```python
from build123d import *

# Parameters (mm, degrees)
BOSS_EXTRUDE1_DEPTH   = 10
M8_TAPPED_HOLE1_D     = 6.8
M8_TAPPED_HOLE1_DEPTH = 14
M8_TAPPED_HOLE1_TIP   = 2.042926105
M5_TAPPED_HOLE1_D     = 4.2
M5_TAPPED_HOLE1_DEPTH = 12
M5_TAPPED_HOLE1_TIP   = 1.2618073


with BuildPart() as part:
    # Sketch1 → Boss-Extrude1 (new, symmetric)
    with BuildSketch(Plane(origin=(0, 0, 0), x_dir=(0, 0, -1), z_dir=(1, 0, 0))):
        Polygon((12, 10), (-12, 10), (-12, 0), (-22, 0), (-22, 32), (22, 32), (22, 0), (12, 0), align=None)
    extrude(amount=BOSS_EXTRUDE1_DEPTH, both=True)

    # M8 Tapped Hole1
    with Locations(Plane(origin=(10, 0, 0), x_dir=(0, 0, -1), z_dir=(1, 0, 0))):
        with Locations((0, 18)):
            Hole(M8_TAPPED_HOLE1_D / 2, depth=M8_TAPPED_HOLE1_DEPTH)
            with Locations((0, 0, -(M8_TAPPED_HOLE1_DEPTH + M8_TAPPED_HOLE1_TIP / 2))):  # 118° drill point
                Cone(0, M8_TAPPED_HOLE1_D / 2, M8_TAPPED_HOLE1_TIP, mode=Mode.SUBTRACT)

    # M5 Tapped Hole1
    with Locations(Plane(origin=(0, 0, 0), x_dir=(-1, 0, 0), z_dir=(0, -1, 0))):
        with Locations((0, 17), (0, -17)):
            Hole(M5_TAPPED_HOLE1_D / 2, depth=M5_TAPPED_HOLE1_DEPTH)
            with Locations((0, 0, -(M5_TAPPED_HOLE1_DEPTH + M5_TAPPED_HOLE1_TIP / 2))):  # 118° drill point
                Cone(0, M5_TAPPED_HOLE1_D / 2, M5_TAPPED_HOLE1_TIP, mode=Mode.SUBTRACT)


solid = part.part
```
Input: part model. Units: mm. Frame: model coordinates. A direction names the side the tool comes from. Give positions to 0.01 mm unless a question says otherwise; leave off trailing zeros. Order: outer loops, then holes, each group sorted by start corner. A loop starts at its lowest first (then second) coordinate and runs counter-clockwise, first axis right, second up. Notation, with made-up numbers: M 16,23 L 54,23 A21 cw 54,43 Z; hole C 15.5,56 d2. An arc over 180 degrees is marked long. Return JSON: item names as keys, results as strings.
Item 1: Pull-direction query (Y, two-part tool) for faces 4 (the conical face through (-5.688, 18.498, -0.317)), 5 (the conical face through (-0.2, 13.04, -17.31)), 6 (the cylindrical face through (1.13, 6.08, -18.77)), 7 (the cylindrical face through (2.9, 14.68, -0.74)); classes: +Y half, -Y half, draft (parallel to the pull), parting line (faces both ways), or undercut.
Solutions:
{"face 4": "undercut", "face 5": "-Y half", "face 6": "draft", "face 7": "undercut"}
Item 2: Cut plane A-A (y = 7). Return loops of the section in (x, z).
Solutions:
{"outline": "M -10,-22 L 10,-22 L 10,-12 L -10,-12 Z; M -10,12 L 10,12 L 10,22 L -10,22 Z; hole C 0,-17 d4.2; hole C 0,17 d4.2"}
Item 3: Cut plane B-B (x = 6.5). Return loops of the section in (y, z), then the cut area to 3 significant figures.
Solutions:
{"outline": "M 0,-22 L 32,-22 L 32,22 L 0,22 L 0,12 L 10,12 L 10,-12 L 0,-12 Z; hole C 18,0 d6.8", "area": "1,130 mm^2"}
Item 4: Access query for faces 1 (the cylindrical face through (-0.273, 6.084, 14.918)), 2 (the flat face through (0, 32, 0)), 3 (the flat face through (0, 5, 12)). Directions: +Z, -Z, +X, -X, +Y, -Y. A direction counts if a zero-diameter tool reaches every point of the face in a straight line with its end or side. Return the directions, or none.
Solutions:
{"face 1": "-Y", "face 2": "+Z, -Z, +X, -X, +Y", "face 3": "+X, -X, -Y"}
Item 5: Ray query, probe 1 along Z at (x, y) = (0, 3.5); probe 2 along Y at (x, z) = (0, 0); probe 3 along X at (y, z) = (7.5, -17). Return the intervals inside material, ascending.
Solutions:
{"probe 1": "-22 to -19.1, -14.9 to -12, 12 to 14.9, 19.1 to 22", "probe 2": "10 to 14.6, 21.4 to 32", "probe 3": "-10 to -2.1, 2.1 to 10"}
Item 6: First-contact query: P1, Ø1.5, axis at x = 5.5, z = -2, coming from the -Y side; P2, Ø6.5, axis at x = 0, z = 17, coming from the -Y side; P3, Ø4, axis at y = 18, z = 0, coming from the +X side. Flat tips, straight axial feed; report the tip coordinate or a pass-through.
Solutions:
{"P1": "y = 10", "P2": "y = 0", "P3": "x = -4.84"}
Item 7: Cut plane C-C (y = 11). Return loops of the section in (x, z).
Solutions:
{"outline": "M -10,-22 L 10,-22 L 10,22 L -10,22 Z; hole C 0,-17 d4.2; hole C 0,17 d4.2"}
